Can you work these out from the model? Positions are in its coordinate system, mm. A direction names the side the tool comes from. Give positions to 0.01 mm unless a question says otherwise; leave off trailing zeros. Loops run counter-clockwise (first coordinate to the right, second up) from the corner with the lowest first, then second, coordinate; pieces in that order, holes last. Notation, with made-up numbers: (88.25, 54) - (135.25, 54) arc R16 cw to (135.25, 77) - close; hole circle Ø8 at (32, 38.25). An arc over 180 degrees is marked (long way). Use a Markdown table: item, result. Add a question column.
```python
from build123d import *

# Parameters (mm, degrees)
SKETCH1_W                                        = 23.9
SKETCH1_H                                        = 40
BOSS_EXTRUDE1_DEPTH                              = 3.4
CUT_EXTRUDE1_DEPTH                               = 30
SKETCH3_W                                        = 14
SKETCH3_H                                        = 30.1
BOSS_EXTRUDE2_DEPTH                              = 1.95
SKETCH4_W                                        = 10.4
SKETCH4_H                                        = 30
CUT_EXTRUDE2_DEPTH                               = 1.55
CUT_EXTRUDE3_REACH                               = 2.95
SKETCH6_W                                        = 10.4
SKETCH6_H                                        = 1.75
CUT_EXTRUDE4_REACH                               = 2.95
SKETCH8_W                                        = 10.4
SKETCH8_H                                        = 1.75
SKETCH9_W                                        = 0.6
SKETCH9_H                                        = 30
CUT_EXTRUDE5_DEPTH                               = 1.8
SKETCH10_W                                       = 0.6
SKETCH10_H                                       = 30
CUT_EXTRUDE6_DEPTH                               = 1.8
SKETCH11_W                                       = 12
SKETCH11_H                                       = 1
BOSS_EXTRUDE3_DEPTH                              = 1.05
SKETCH12_W                                       = 12
SKETCH12_H                                       = 1
BOSS_EXTRUDE4_DEPTH                              = 1.05
CBORE_FOR_M4_HEX_HEAD_MACHINE_SCREW1_D           = 4.5
CBORE_FOR_M4_HEX_HEAD_MACHINE_SCREW1_DEPTH       = 3.8
CBORE_FOR_M4_HEX_HEAD_MACHINE_SCREW1_CBORE_D     = 8.5
CBORE_FOR_M4_HEX_HEAD_MACHINE_SCREW1_CBORE_DEPTH = 2.3
CHAMFER1_SIZE                                    = 0.527
CHAMFER1_SIZE2                                   = 0.913344887
CHAMFER1_PART_2_SIZE                             = 0.527
CHAMFER1_PART_2_SIZE2                            = 0.913344887
CHAMFER1_PART_3_SIZE                             = 0.527
CHAMFER1_PART_3_SIZE2                            = 0.913344887
CHAMFER2_SIZE                                    = 0.2
CHAMFER3_SIZE                                    = 0.577
CHAMFER4_SIZE                                    = 0.913344887
CHAMFER4_SIZE2                                   = 0.527
FILLET1_R                                        = 0.5


with BuildPart() as part:
    # Sketch1 → Boss-Extrude1 (new body)
    with BuildSketch(Plane.XY.offset(7.55)):
        Rectangle(SKETCH1_W, SKETCH1_H)
    extrude(amount=-BOSS_EXTRUDE1_DEPTH)

    # Sketch2 → Cut-Extrude1 (cut)
    with BuildSketch(Plane.XZ.offset(15)):
        with BuildLine():
            Line((7, 7.310697145), (7, 7.55))
            Line((7, 7.55), (6.995, 7.55))
            Line((6.995, 7.55), (6.995, 7.4))
            ThreePointArc((6.995, 7.4), (6.996250978, 7.35527864), (7, 7.310697145))
        make_face()
    extrude(amount=-CUT_EXTRUDE1_DEPTH, mode=Mode.SUBTRACT)

    # Sketch3 → Boss-Extrude2 (add)
    with BuildSketch(Plane.XY.offset(7.55)):
        with Locations((-0.005, 0)):
            Rectangle(SKETCH3_W, SKETCH3_H)
    extrude(amount=BOSS_EXTRUDE2_DEPTH)

    # Sketch4 → Cut-Extrude2 (cut)
    with BuildSketch(Plane(origin=(0, 0, 4.15), x_dir=(-1, 0, 0), z_dir=(0, 0, -1))):
        Rectangle(SKETCH4_W, SKETCH4_H)
    extrude(amount=-CUT_EXTRUDE2_DEPTH, mode=Mode.SUBTRACT)

    # Sketch6 → Cut-Extrude3 (cut, up to next)
    with BuildSketch(Plane.XY.offset(5.1), mode=Mode.PRIVATE) as cut_extrude3_sk1:
        with Locations((0, -15.875)):
            Rectangle(SKETCH6_W, SKETCH6_H)
    cut_extrude3_tool1 = extrude(cut_extrude3_sk1.sketch, amount=-CUT_EXTRUDE3_REACH, mode=Mode.PRIVATE) & part.part
    add(cut_extrude3_tool1.solids().sort_by_distance((0, -15.875, 5.1))[0], mode=Mode.SUBTRACT)

    # Sketch8 → Cut-Extrude4 (cut, up to next)
    with BuildSketch(Plane.XY.offset(5.1), mode=Mode.PRIVATE) as cut_extrude4_sk1:
        with Locations((0, 15.875)):
            Rectangle(SKETCH8_W, SKETCH8_H)
    cut_extrude4_tool1 = extrude(cut_extrude4_sk1.sketch, amount=-CUT_EXTRUDE4_REACH, mode=Mode.PRIVATE) & part.part
    add(cut_extrude4_tool1.solids().sort_by_distance((0, 15.875, 5.1))[0], mode=Mode.SUBTRACT)

    # Sketch9 → Cut-Extrude5 (cut)
    with BuildSketch(Plane(origin=(-5.2, 0, 0), x_dir=(0, 0, -1), z_dir=(1, 0, 0))):
        with Locations((-5.4, 0)):
            Rectangle(SKETCH9_W, SKETCH9_H)
    extrude(amount=-CUT_EXTRUDE5_DEPTH, mode=Mode.SUBTRACT)

    # Sketch10 → Cut-Extrude6 (cut)
    with BuildSketch(Plane.ZY.offset(-5.2)):
        with Locations((5.4, 0)):
            Rectangle(SKETCH10_W, SKETCH10_H)
    extrude(amount=-CUT_EXTRUDE6_DEPTH, mode=Mode.SUBTRACT)

    # Sketch11 → Boss-Extrude3 (add)
    with BuildSketch(Plane.XY.offset(7.55)):
        with Locations((0, 19.5)):
            Rectangle(SKETCH11_W, SKETCH11_H)
    extrude(amount=BOSS_EXTRUDE3_DEPTH)

    # Sketch12 → Boss-Extrude4 (add)
    with BuildSketch(Plane.XY.offset(7.55)):
        with Locations((0, -19.5)):
            Rectangle(SKETCH12_W, SKETCH12_H)
    extrude(amount=BOSS_EXTRUDE4_DEPTH)

    # CBORE for M4 Hex Head Machine Screw1
    with Locations(Plane(origin=(0, 0, 5.7), x_dir=(-1, 0, 0), z_dir=(0, 0, -1))):
        with Locations((0, 10), (0, -10)):
            CounterBoreHole(CBORE_FOR_M4_HEX_HEAD_MACHINE_SCREW1_D / 2, CBORE_FOR_M4_HEX_HEAD_MACHINE_SCREW1_CBORE_D / 2, CBORE_FOR_M4_HEX_HEAD_MACHINE_SCREW1_CBORE_DEPTH, depth=CBORE_FOR_M4_HEX_HEAD_MACHINE_SCREW1_DEPTH)

    # Chamfer1
    chamfer1_edges = [part.edges().sort_by_distance(p)[0] for p in [
        (-11.95, 20, 5.85),
    ]]
    chamfer1_side = [part.faces().sort_by_distance(p)[0] for p in [
        (0, 20, 6.148689538),
    ]]
    chamfer(chamfer1_edges, length=CHAMFER1_SIZE, length2=CHAMFER1_SIZE2, reference=chamfer1_side[0])

    # Chamfer1 part 2
    chamfer1_part_2_edges = [part.edges().sort_by_distance(p)[0] for p in [
        (11.95, -20, 5.85),
    ]]
    chamfer1_part_2_side = [part.faces().sort_by_distance(p)[0] for p in [
        (0, -20, 6.148689538),
    ]]
    chamfer(chamfer1_part_2_edges, length=CHAMFER1_PART_2_SIZE, length2=CHAMFER1_PART_2_SIZE2, reference=chamfer1_part_2_side[0])

    # Chamfer1 part 3
    chamfer1_part_3_edges = [part.edges().sort_by_distance(p)[0] for p in [
        (-11.95, -20, 5.85),
    ]]
    chamfer1_part_3_side = [part.faces().sort_by_distance(p)[0] for p in [
        (-11.95, 0, 5.85),
    ]]
    chamfer(chamfer1_part_3_edges, length=CHAMFER1_PART_3_SIZE, length2=CHAMFER1_PART_3_SIZE2, reference=chamfer1_part_3_side[0])

    # Chamfer2
    chamfer2_edges = [part.edges().sort_by_distance(p)[0] for p in [
        (-2.25, -10, 8),
        (-2.25, 10, 8),
    ]]
    chamfer(chamfer2_edges, length=CHAMFER2_SIZE)

    # Chamfer3
    chamfer3_edges = [part.edges().sort_by_distance(p)[0] for p in [
        (11.95, 0.456672444, 7.55),
        (11.95, 0.456672444, 4.15),
        (-11.95, -0.193172444, 4.15),
        (-11.95, -0.193172444, 7.55),
    ]]
    chamfer(chamfer3_edges, length=CHAMFER3_SIZE)

    # Chamfer4
    chamfer4_edges = [part.edges().sort_by_distance(p)[0] for p in [
        (11.95, 20, 5.85),
    ]]
    chamfer4_side = [part.faces().sort_by_distance(p)[0] for p in [
        (11.95, 0.456672444, 5.85),
    ]]
    chamfer(chamfer4_edges, length=CHAMFER4_SIZE, length2=CHAMFER4_SIZE2, reference=chamfer4_side[0])

    # Fillet1
    fillet1_edges = [part.edges().sort_by_distance(p)[0] for p in [
        (6.995, 0, 9.5),
        (-7.005, 0, 9.5),
    ]]
    fillet(fillet1_edges, radius=FILLET1_R)


solid = part.part
```
1. Suppose I cut it at D-D (x = -10). List the corners of the cut face in (y, z) for me, and give its area (3 significant figures).
2. On a 3-axis mill with a long thin cutter (end or side, diameter ignored), from which of +Z, -Z, +X, -X, +Y, -Y can I reach the whole of each face in a straight line? I mean faces 4 (the face through (6, 0, 5.1)), 5 (the face through (0, 19, 8)), 6 (the face through (0, 16, 5.1)). Say none if no direction works.
3. Suppose I cut it at B-B (x = 0). State how many separate pieces and enclosed holes the cut face has, and give its area (3 significant figures).
4. If we mould it in two halves opening along Y, with no side actions, what happens to faces 1 (the face through (5.2, -0.2, 4.6)), 2 (the face through (-11.69, 19.54, 5.87)), 3 (the face through (-0.1, -19.5, 8.6))? For each: released by +Y, released by -Y, zero draft, split by the parting line, or undercut.
5. Suppose I cut it at C-C (y = 3.5). List the corners of the cut face in (x, z) for me (3 decimals).
6. Will these pins go through, and if not, where does the flat tip stop? P1, Ø0.8, axis at y = -7.5, z = 8, coming from the +X side (3 decimals); P2, Ø1.1, axis at x = -1.5, y = -19.5, coming from the +Z side; P3, Ø1, axis at y = 5.5, z = 8, coming from the +X side; P4, Ø4, axis at x = 0, y = 10, coming from the -Z side.
7. Please list where these lines run through material, in increasing order: line 1 along Y through (x, z) = (0, 7.05); line 2 along Y through (x, z) = (5.75, 8.45); line 3 along Z through (x, y) = (6.25, 3.5). Write a range as [from, to].
Results below:
| question | item | result |
|---|---|---|
| 1 | outline | (-20, 4.15) - (20, 4.15) - (20, 7.55) - (-20, 7.55) - close |
| 1 | area | 136 mm² |
| 2 | face 4 | none |
| 2 | face 5 | +Z, +X, -X |
| 2 | face 6 | -Z |
| 3 | separate pieces | 3 |
| 3 | enclosed holes | 0 |
| 3 | area | 94.3 mm² |
| 4 | face 1 | undercut |
| 4 | face 2 | released by +Y |
| 4 | face 3 | zero draft |
| 5 | outline | (-11.95, 4.727) - (-11.373, 4.15) - (-5.2, 4.15) - (-5.2, 5.1) - (-7, 5.1) - (-7, 5.7) - (7, 5.7) - (7, 5.1) - (5.2, 5.1) - (5.2, 4.15) - (11.373, 4.15) - (11.95, 4.727) - (11.95, 6.973) - (11.373, 7.55) - (7, 7.55) - (7, 7.311) arc R0.8 cw to (6.995, 7.4) - (6.995, 9) arc R0.5 ccw to (6.495, 9.5) - (-6.505, 9.5) arc R0.5 ccw to (-7.005, 9) - (-7.005, 7.55) - (-11.373, 7.55) - (-11.95, 6.973) - close |
| 6 | P1 | x = 6.995 |
| 6 | P2 | z = 8.6 |
| 6 | P3 | x = 11.42 |
| 6 | P4 | through |
| 7 | line 1 | [-20, -14.25], [-5.75, 5.75], [14.25, 20] |
| 7 | line 2 | [-20, -19], [-15.05, 15.05], [19, 20] |
| 7 | line 3 | [4.15, 5.1], [5.7, 9.5] |
